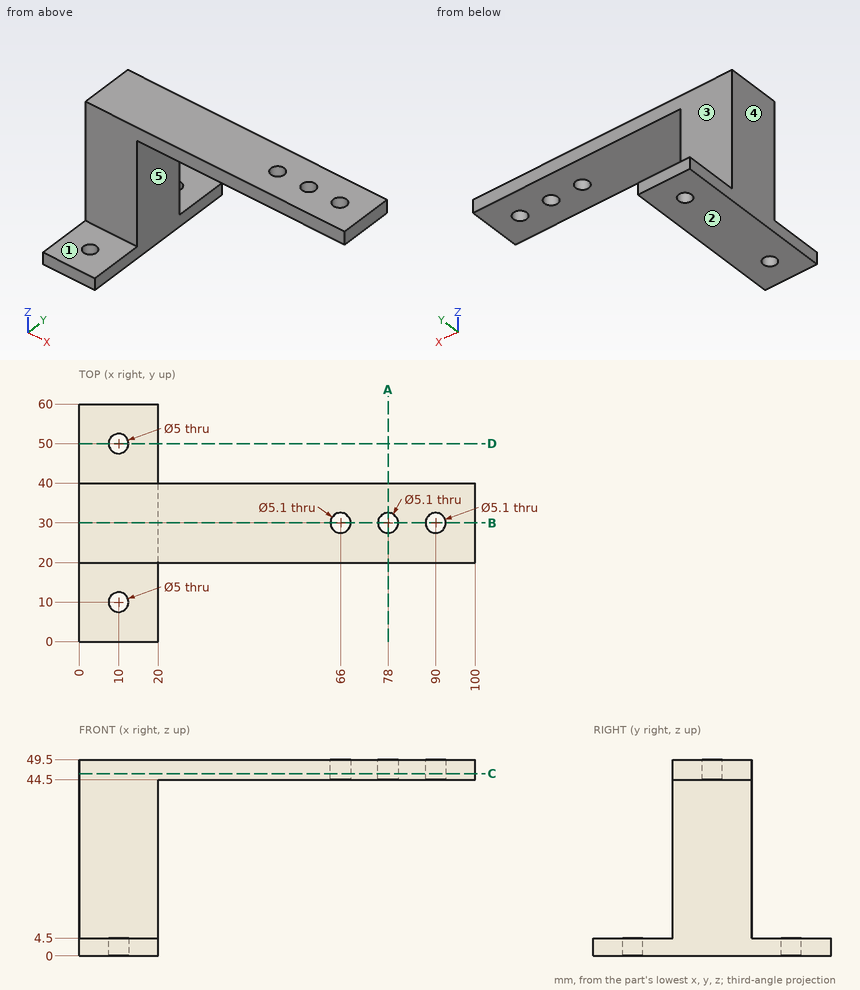
Geometry check sheet. Reference: drawing and pictorial views, mm from the part's lowest x, y, z. A direction names the side the tool comes from. Round coordinates to 2 decimals unless told otherwise and drop trailing zeros. Loops run counter-clockwise (first coordinate to the right, second up) from the corner with the lowest first, then second, coordinate; pieces in that order, holes last.
1. Sectioned sample at D-D on y = 50. Record the boundary of the cut face in (x, z).
2. Sectioned sample at A-A on x = 78. Record the boundary of the cut face in (y, z).
3. Sectioned sample at B-B on y = 30. Record the boundary of the cut face in (x, z).
4. Scan lines: probe 1 along Y at (x, z) = (90, 48.35); probe 2 along X at (y, z) = (28.5, 43); probe 3 along Z at (x, y) = (87, 29). Record each from-to range of solid material in increasing order.
5. Set-up check for the marked faces 1, 2, 3, 4 and 5: record each of +Z, -Z, +X, -X, +Y, -Y from which the full face is reachable in a straight line by a thin tool's end or side.
6. Gauge pin test, flat ends, axial feed: pin 1 Ø2 at (y, z) = (33, 11) entering from -X; pin 2 Ø22.5 at (x, z) = (29.5, 34) entering from -Y; pin 3 Ø6 at (x, y) = (42.5, 32) entering from -Z; pin 4 Ø1.5 at (x, z) = (60, 44) entering from +Y. Record the tip position at first contact, or that the pin passes through.
7. Sectioned sample at C-C on z = 46. Record the boundary of the cut face in (x, y), and give its area (3 significant figures).
Recorded:
1. outline: (0, 0) - (7.5, 0) - (7.5, 4.5) - (0, 4.5) - close; (12.5, 0) - (20, 0) - (20, 4.5) - (12.5, 4.5) - close
2. outline: (20, 44.5) - (27.45, 44.5) - (27.45, 49.5) - (20, 49.5) - close; (32.55, 44.5) - (40, 44.5) - (40, 49.5) - (32.55, 49.5) - close
3. outline: (0, 0) - (20, 0) - (20, 44.5) - (63.45, 44.5) - (63.45, 49.5) - (0, 49.5) - close; (68.55, 44.5) - (75.45, 44.5) - (75.45, 49.5) - (68.55, 49.5) - close; (80.55, 44.5) - (87.45, 44.5) - (87.45, 49.5) - (80.55, 49.5) - close; (92.55, 44.5) - (100, 44.5) - (100, 49.5) - (92.55, 49.5) - close
4. probe 1: y = 20 to 27.45, 32.55 to 40
4. probe 2: x = 0 to 20
4. probe 3: z = 44.5 to 49.5
5. face 1: +Z, +X, -X, -Y
5. face 2: -Z, +X, -X, +Y, -Y
5. face 3: +Z, +X, -X, +Y
5. face 4: +Z, -Z, -X, +Y, -Y
5. face 5: -Z, +X, +Y, -Y
6. pin 1: stops at x = 0
6. pin 2: stops at y = 20
6. pin 3: stops at z = 44.5
6. pin 4: stops at y = 40
7. outline: (0, 20) - (100, 20) - (100, 40) - (0, 40) - close; hole circle Ø5.1 at (66, 30); hole circle Ø5.1 at (78, 30); hole circle Ø5.1 at (90, 30)
7. area: 1,940 mm2
